from build123d import *

# Parameters (mm, degrees)
BOSS_EXTRUDE1_DEPTH     = 308
CUT_EXTRUDE1_START      = -62.5
SKETCH4_R               = 3.5
CUT_EXTRUDE1_DEPTH      = 2.111341
CIRPATTERN2_COUNT       = 2
CIRPATTERN2_ANGLE       = 80
MIRROR1_START           = -62.5
MIRROR1_COPY_1_SKETCH_R = 3.5
MIRROR1_COPY_1_DEPTH    = 2.111341
MIRROR1_COPY_2_SKETCH_R = 3.5
MIRROR1_COPY_2_DEPTH    = 2.111341
SKETCH5_R               = 3.5
CUT_EXTRUDE2_DEPTH      = 5


with BuildPart() as part:
    # Sketch3 → Boss-Extrude1 (new body)
    with BuildSketch(Plane(origin=(0, 0, 0), x_dir=(1, 0, 0), z_dir=(0, 1, 0))):
        with BuildLine():
            Line((0, -60.49), (0, -60.75))
            Line((0, -60.75), (1.5, -60.75))
            Line((1.5, -60.75), (1.5, -62.25))
            Line((1.5, -62.25), (0, -62.25))
            Line((0, -62.25), (0, -62.5))
            ThreePointArc((0, -62.5), (-62.5, 0), (0, 62.5))
            Line((0, 62.5), (0, 62.25))
            Line((0, 62.25), (1.5, 62.25))
            Line((1.5, 62.25), (1.5, 60.75))
            Line((1.5, 60.75), (0, 60.75))
            Line((0, 60.75), (0, 60.49))
            ThreePointArc((0, 60.49), (-60.49, 0), (0, -60.49))
        make_face()
    extrude(amount=BOSS_EXTRUDE1_DEPTH)

    # Sketch4 → Cut-Extrude1 (cut)
    with BuildSketch(Plane(origin=(0, 0, 0), x_dir=(0, 0, -1), z_dir=(1, 0, 0)).offset(CUT_EXTRUDE1_START)):
        with Locations((0, 10)):
            Circle(SKETCH4_R)
    cut_extrude1 = extrude(amount=CUT_EXTRUDE1_DEPTH, mode=Mode.SUBTRACT)

    # CirPattern2: Cut-Extrude1 ×2 about axis
    cirpattern2_axis = Axis((0, 0, 0), (0, 1, 0))
    for i in range(1, CIRPATTERN2_COUNT):
        add(cut_extrude1.rotate(cirpattern2_axis, i * CIRPATTERN2_ANGLE / (CIRPATTERN2_COUNT - 1)), mode=Mode.SUBTRACT)

    # Mirror1 copy 1 sketch → Mirror1 copy 1 (cut)
    with BuildSketch(Plane(origin=(0, 0, 0), x_dir=(-0.984807753, 0, 0.173648178), z_dir=(0.173648178, 0, 0.984807753)).offset(MIRROR1_START)):
        with Locations((0, -10)):
            Circle(MIRROR1_COPY_1_SKETCH_R)
    extrude(amount=MIRROR1_COPY_1_DEPTH, mode=Mode.SUBTRACT)

    # Mirror1 copy 2 sketch → Mirror1 copy 2 (cut)
    with BuildSketch(Plane(origin=(0, 0, 0), x_dir=(0, 0, 1), z_dir=(1, 0, 0)).offset(MIRROR1_START)):
        with Locations((0, -10)):
            Circle(MIRROR1_COPY_2_SKETCH_R)
    extrude(amount=MIRROR1_COPY_2_DEPTH, mode=Mode.SUBTRACT)

    # Sketch5 → Cut-Extrude2 (cut, symmetric)
    with BuildSketch(Plane(origin=(0, 0, -62.5), x_dir=(-1, 0, 0), z_dir=(0, 0, -1))):
        with Locations((5, 288)):
            Circle(SKETCH5_R)
    cut_extrude2 = extrude(amount=CUT_EXTRUDE2_DEPTH, both=True, mode=Mode.SUBTRACT)

    # Mirror2: Cut-Extrude2 across plane
    add(cut_extrude2.mirror(Plane.XY), mode=Mode.SUBTRACT)


solid = part.part
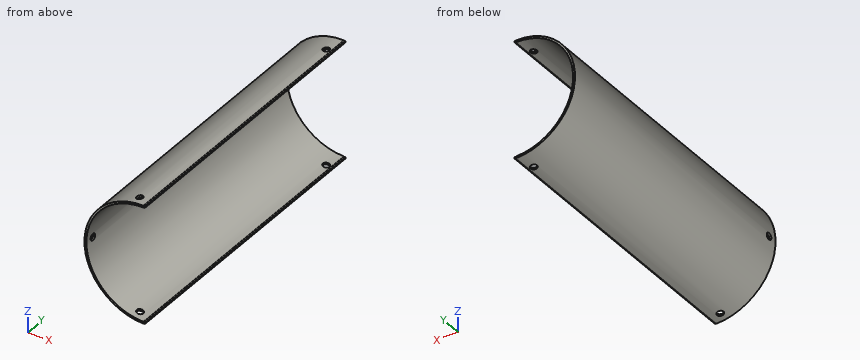
Can you work these out from the model? Positions are in its coordinate system, mm. Give positions to 0.01 mm unless a question says otherwise; leave off trailing zeros. Order: outer loops, then holes, each group sorted by start corner. A loop starts at its lowest first (then second) coordinate and runs counter-clockwise, first axis right, second up. Notation, with made-up numbers: M -22.75,78 L -7.75,78 A13 cw -7.75,95 Z; hole C 62.5,33.5 d4. An arc over 180 degrees is marked long. One line per item, written item: value.
Item 1: If we section it at D-D on y = 175.5: Write out the boundary of the cut face in (x, z), and give its area (3 significant figures).
Verdict:
outline: M 0,-62.5 L 0,-62.25 L 1.5,-62.25 L 1.5,-60.75 L 0,-60.75 L 0,-60.49 A60.49 cw 0,60.49 L 0,60.75 L 1.5,60.75 L 1.5,62.25 L 0,62.25 L 0,62.5 A62.5 ccw Z
area: 393 mm2
Item 2: For pin 1 (1 mm diameter, centred on x = -56, y = 104.5, fed in from -Z); pin 2 (2 mm diameter, centred on y = 276.5, z = -15.5, fed in from +X); pin 3 (0.8 mm diameter, centred on x = 1, y = 98, fed in from +Z), each with a flat end and sliding along its axis, tell me the tip position at first contact or that it passes through.
Verdict:
pin 1: z = -28.74
pin 2: x = -58.2
pin 3: z = 62.25
Item 3: Please list where these lines run through material, in increasing order: line 1 (Y direction, x = -60.9, z = 0); line 2 (Y direction, x = -5, z = 61.35); line 3 (Z direction, x = -56, y = 89).
Verdict:
line 1: 0 to 6.5, 13.5 to 308
line 2: 0 to 284.5, 291.5 to 308
line 3: -27.75 to -22.87, 22.87 to 27.75
Item 4: If we section it at B-B on x = -40.5: Write out the boundary of the cut face in (y, z).
Verdict:
outline: M 0,-47.6 L 308,-47.6 L 308,-44.93 L 0,-44.93 Z; M 0,44.93 L 308,44.93 L 308,47.6 L 0,47.6 Z
Item 5: If we section it at C-C on y = 10: Write out the boundary of the cut face in (x, z).
Verdict:
outline: M -62.4,-3.5 A62.5 ccw -14.28,-60.85 L -13.93,-58.86 A60.49 cw -60.39,-3.5 Z; M -62.4,3.5 L -60.39,3.5 A60.49 cw -13.93,58.86 L -14.28,60.85 A62.5 ccw Z; M -7.39,-62.06 A62.5 ccw 0,-62.5 L 0,-62.25 L 1.5,-62.25 L 1.5,-60.75 L 0,-60.75 L 0,-60.49 A60.49 cw -7.04,-60.08 Z; M -7.39,62.06 L -7.04,60.08 A60.49 cw 0,60.49 L 0,60.75 L 1.5,60.75 L 1.5,62.25 L 0,62.25 L 0,62.5 A62.5 ccw Z
Item 6: If we section it at A-A on z = 0: Write out the boundary of the cut face in (x, y), and give its area (3 significant figures).
Verdict:
outline: M -62.5,0 L -60.49,0 L -60.49,6.5 L -62.5,6.5 Z; M -62.5,13.5 L -60.49,13.5 L -60.49,308 L -62.5,308 Z
area: 605 mm2
